Build history of the part. All positions in model axes, mm. Face numbers are marked on the shaded views. A direction names the side the tool comes from. Round coordinates to 2 decimals unless told otherwise and drop trailing zeros. Write each loop counter-clockwise with the first axis right and the second up, starting at its lowest first coordinate (ties: lowest second). Pieces come first, ordered by that corner, then holes.
1) Which spindle directions (+Z, -Z, +X, -X, +Y, -Y) get a long thin tool onto all of the face, cutting with end or side? Do the marked faces 1, 2, 3 and 4. Say none if no direction does.
2) Flat gauge pins, fed straight in: pin 1 (12 mm diameter, centred on y = 29, z = 0, fed in from -X); pin 2 (12 mm diameter, centred on x = 56, z = -1.5, fed in from -Y); pin 3 (10 mm diameter, centred on x = 54.5, z = 12, fed in from -Y); pin 4 (3.5 mm diameter, centred on y = 41, z = -1.5, fed in from +X). Where does each tip first touch, or does it go through?
3) Saw through at C-C (x = 31). Write the cut outline in (y, z).
4) Saw through at D-D (z = 0). State how many separate pieces and enclosed holes the cut face has, plus the area to 3 significant figures.
5) Wall check: probe 1 along X at (y, z) = (20, 0); probe 2 along Z at (x, y) = (31, 34.5); probe 3 along X at (y, z) = (25, 0). Give the ranges that are in metal, low to high.
6) Saw through at B-B (y = 46). Write the cut outline in (x, z), plus the area to 3 significant figures.
7) Pull direction Z, two halves, no side cores. Call the marked faces 5, 6, 7 and 8: +Z half, -Z half, draft (parallel to the pull), parting line (faces both ways), or undercut.
8) Saw through at A-A (y = 7). Write the cut outline in (x, z), plus the area to 3 significant figures.
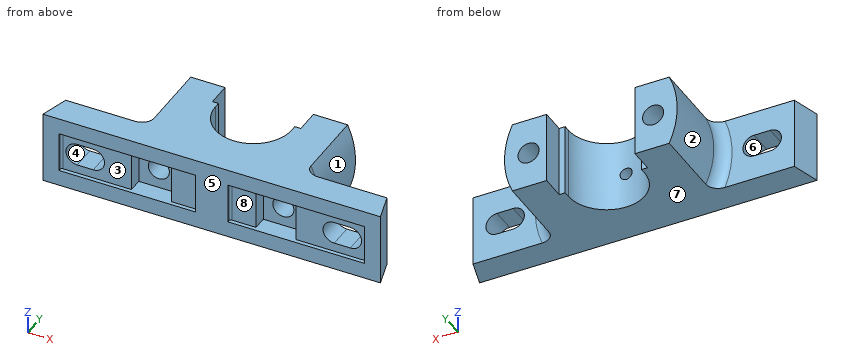
from build123d import *

# Parameters (mm, degrees)
BOSS_EXTRUDE1_DEPTH = 18
BOSS_EXTRUDE2_DEPTH = 41
CUT_EXTRUDE1_DEPTH  = 12
FILLET1_R           = 6
CUT_EXTRUDE2_DEPTH  = 37.0000001
SKETCH7_R           = 5.25
CUT_EXTRUDE3_DEPTH  = 46
SKETCH10_W          = 68
SKETCH10_H          = 20
CUT_EXTRUDE4_DEPTH  = 2
FILLET2_R           = 1
SKETCH11_W          = 20
SKETCH11_H          = 20
CUT_EXTRUDE5_DEPTH  = 9
SKETCH15_R          = 3
CUT_EXTRUDE6_DEPTH  = 10


with BuildPart() as part:
    # Sketch2 → Boss-Extrude1 (new body, symmetric)
    with BuildSketch(Plane.XY):
        Polygon((-84, 0), (84, 0), (80, 14), (-80, 14), align=None)
    extrude(amount=BOSS_EXTRUDE1_DEPTH, both=True)

    # Sketch3 → Boss-Extrude2 (add)
    with BuildSketch(Plane(origin=(0, 14, 0), x_dir=(1, 0, 0), z_dir=(0, 1, 0))):
        with BuildLine():
            Line((-39.05124838, 18), (39.05124838, 18))
            ThreePointArc((39.05124838, 18), (43, 0), (39.05124838, -18))
            Line((39.05124838, -18), (-39.05124838, -18))
            ThreePointArc((-39.05124838, -18), (-43, 0), (-39.05124838, 18))
        make_face()
    extrude(amount=BOSS_EXTRUDE2_DEPTH)

    # Sketch4 → Cut-Extrude1 (cut)
    with BuildSketch(Plane(origin=(0, 14, 0), x_dir=(1, 0, 0), z_dir=(0, 1, 0))):
        with BuildLine():
            Line((60, 5.595094271), (68, 5.595094271))
            ThreePointArc((68, 5.595094271), (73.595094271, 0), (68, -5.595094271))
            Line((68, -5.595094271), (60, -5.595094271))
            ThreePointArc((60, -5.595094271), (54.404905729, 0), (60, 5.595094271))
        make_face()
        with BuildLine():
            Line((-60, 5.595094271), (-68, 5.595094271))
            ThreePointArc((-68, 5.595094271), (-73.595094271, 0), (-68, -5.595094271))
            Line((-68, -5.595094271), (-60, -5.595094271))
            ThreePointArc((-60, -5.595094271), (-54.404905729, 0), (-60, 5.595094271))
        make_face()
    extrude(amount=-CUT_EXTRUDE1_DEPTH, mode=Mode.SUBTRACT)

    # Fillet1
    fillet1_edges = [part.edges().sort_by_distance(p)[0] for p in [
        (43, 14, 0),
        (-43, 14, 0),
    ]]
    fillet(fillet1_edges, radius=FILLET1_R)

    # Sketch5 → Cut-Extrude2 (cut, through all)
    with BuildSketch(Plane.XY.offset(18)):
        with BuildLine():
            Line((22, 55), (22, 43))
            Line((22, 43), (19, 43))
            Line((19, 43), (19, 40))
            ThreePointArc((19, 40), (0, 21), (-19, 40))
            Line((-19, 40), (-19, 43))
            Line((-19, 43), (-22, 43))
            Line((-22, 43), (-22, 55))
            Line((-22, 55), (22, 55))
        make_face()
    extrude(amount=-CUT_EXTRUDE2_DEPTH, mode=Mode.SUBTRACT)

    # Sketch7 → Cut-Extrude3 (cut)
    with BuildSketch(Plane(origin=(0, 55, 0), x_dir=(1, 0, 0), z_dir=(0, 1, 0))):
        with Locations((31, 0)):
            Circle(SKETCH7_R)
        with Locations((-31, 0)):
            Circle(SKETCH7_R)
    extrude(amount=-CUT_EXTRUDE3_DEPTH, mode=Mode.SUBTRACT)

    # Sketch10 → Cut-Extrude4 (cut)
    with BuildSketch(Plane.XZ):
        with Locations((42, 0)):
            Rectangle(SKETCH10_W, SKETCH10_H)
        with Locations((-42, 0)):
            Rectangle(SKETCH10_W, SKETCH10_H)
    extrude(amount=-CUT_EXTRUDE4_DEPTH, mode=Mode.SUBTRACT)

    # Fillet2
    fillet2_edges = [part.edges().sort_by_distance(p)[0] for p in [
        (76, 2, 0),
        (8, 2, 0),
        (-8, 2, 0),
        (-76, 2, 0),
    ]]
    fillet(fillet2_edges, radius=FILLET2_R)

    # Sketch11 → Cut-Extrude5 (cut)
    with BuildSketch(Plane.XZ):
        with Locations((31, 0)):
            Rectangle(SKETCH11_W, SKETCH11_H)
        with Locations((-31, 0)):
            Rectangle(SKETCH11_W, SKETCH11_H)
    extrude(amount=-CUT_EXTRUDE5_DEPTH, mode=Mode.SUBTRACT)

    # Sketch15 → Cut-Extrude6 (cut)
    with BuildSketch(Plane(origin=(0, 25, 0), x_dir=(-1, 0, 0), z_dir=(0, -1, 0))):
        Circle(SKETCH15_R)
    extrude(amount=CUT_EXTRUDE6_DEPTH, mode=Mode.SUBTRACT)


solid = part.part
Evaluation:
1. face 1: +X, +Y
1. face 2: -X, +Y
1. face 3: -Y
1. face 4: +Y, -Y
2. pin 1: stops at x = -43
2. pin 2: stops at y = 2
2. pin 3: stops at y = 0
2. pin 4: stops at x = 43
3. outline: (0, -18) - (55, -18) - (55, -5.25) - (9, -5.25) - (9, -10) - (0, -10) - close; (0, 10) - (9, 10) - (9, 5.25) - (55, 5.25) - (55, 18) - (0, 18) - close
4. separate pieces: 5
4. enclosed holes: 0
4. area: 2,610 mm2
5. probe 1: x = -43 to -36.25, -25.75 to -3, 3 to 25.75, 36.25 to 43
5. probe 2: z = -18 to -5.25, 5.25 to 18
5. probe 3: x = -43 to -36.25, -25.75 to -11.66, 11.66 to 25.75, 36.25 to 43
6. outline: (-39.05, -18) - (-22, -18) - (-22, 18) - (-39.05, 18) arc R43 ccw to start; (22, -18) - (39.05, -18) arc R43 ccw to (39.05, 18) - (22, 18) - close; hole circle Ø10.5 at (-31, 0); hole circle Ø10.5 at (31, 0)
6. area: 1,250 mm2
7. face 5: draft
7. face 6: undercut
7. face 7: -Z half
7. face 8: undercut
8. outline: (-82, -18) - (82, -18) - (82, 18) - (-82, 18) - close; hole (-68, -5.6) - (-60, -5.6) arc R5.6 ccw to (-60, 5.6) - (-68, 5.6) arc R5.6 ccw to start; hole (-41, -10) - (-21, -10) - (-21, 10) - (-41, 10) - close; hole (21, -10) - (41, -10) - (41, 10) - (21, 10) - close; hole (60, -5.6) - (68, -5.6) arc R5.6 ccw to (68, 5.6) - (60, 5.6) arc R5.6 ccw to start
8. area: 4,730 mm2
